Geometry check sheet. Reference: the model listing, model coordinates, mm. A direction names the side the tool comes from. Coordinates: 2 decimals unless noted, no trailing zeros. Write each loop counter-clockwise with the first axis right and the second up, starting at its lowest first coordinate (ties: lowest second). Pieces come first, ordered by that corner, then holes. Notation, with made-up numbers: (-2, -32.75) -> (36, -32.75) arc R24 cw to (36, 4.25) -> close; hole circle Ø6 at (87.25, 2). An arc over 180 degrees is marked (long way). Put each result on its own line as item: value. Start each with the question number.
from build123d import *
from OCP.BRepFilletAPI import BRepFilletAPI_MakeChamfer

# Parameters (mm, degrees)
SKETCH1_W           = 42
SKETCH1_H           = 130
BOSS_EXTRUDE1_DEPTH = 3
SKETCH2_W           = 27
SKETCH2_H           = 100
CUT_EXTRUDE1_DEPTH  = 3
BOSS_EXTRUDE2_DEPTH = 10
CHAMFER1_SIZE       = 43.314758743
CHAMFER1_SIZE_2     = 10
SKETCH5_R           = 1.75
CUT_EXTRUDE2_DEPTH  = 10
SKETCH6_W           = 7.5
SKETCH6_H           = 3
BOSS_EXTRUDE3_DEPTH = 10
LPATTERN1_COUNT     = 2
LPATTERN1_PITCH     = 10
FILLET1_R           = 10


with BuildPart() as part:
    # Sketch1 → Boss-Extrude1 (new body)
    with BuildSketch(Plane.XY):
        Rectangle(SKETCH1_W, SKETCH1_H)
    extrude(amount=BOSS_EXTRUDE1_DEPTH)

    # Sketch2 → Cut-Extrude1 (cut)
    with BuildSketch(Plane.XY.offset(3)):
        with Locations((0, -65)):
            Rectangle(SKETCH2_W, SKETCH2_H)
    extrude(amount=-CUT_EXTRUDE1_DEPTH, mode=Mode.SUBTRACT)

    # Sketch3 → Boss-Extrude2 (add)
    with BuildSketch(Plane(origin=(0, 0, 0), x_dir=(-1, 0, 0), z_dir=(0, 0, -1))):
        Polygon((-21, -65), (-13.5, -65), (-13.5, -62), (-13.5, -17), (-15.5, -17), (-15.5, -62), (-21, -62), align=None)
        Polygon((13.5, -65), (21, -65), (21, -62), (15.5, -62), (15.5, -17), (13.5, -17), (13.5, -62), align=None)
    extrude(amount=BOSS_EXTRUDE2_DEPTH)

    # Chamfer1
    chamfer1_edges_1 = [part.edges().sort_by_distance(p)[0] for p in [
        (-14.5, -17, -10),
    ]]
    chamfer1_side_1 = [part.faces().sort_by_distance(p)[0] for p in [
        (-14.5, -17.2, -10),
    ]]
    chamfer1_edges_2 = [part.edges().sort_by_distance(p)[0] for p in [
        (14.5, -17, -10),
    ]]
    chamfer1_side_2 = [part.faces().sort_by_distance(p)[0] for p in [
        (14.5, -17.2, -10),
    ]]
    chamfer1 = BRepFilletAPI_MakeChamfer(part.part.solid().wrapped)
    for e in chamfer1_edges_1:
        chamfer1.Add(CHAMFER1_SIZE - 0.0001, CHAMFER1_SIZE_2 - 0.0001, e.wrapped, chamfer1_side_1[0].wrapped)
    for e in chamfer1_edges_2:
        chamfer1.Add(CHAMFER1_SIZE - 0.0001, CHAMFER1_SIZE_2 - 0.0001, e.wrapped, chamfer1_side_2[0].wrapped)
    add(Compound.cast(chamfer1.Shape()), mode=Mode.REPLACE)  # a hair under: the kernel refuses the full size

    # Sketch5 → Cut-Extrude2 (cut)
    with BuildSketch(Plane.XZ.offset(65)):
        with Locations(Location((-17.5, -4.36859694, 0), (0, 0, 270))):
            Circle(SKETCH5_R)
        with Locations(Location((17.5, -4.36859694, 0), (0, 0, 270))):
            Circle(SKETCH5_R)
    cut_extrude2 = extrude(amount=-CUT_EXTRUDE2_DEPTH, mode=Mode.SUBTRACT)

    # Sketch6 → Boss-Extrude3 (add)
    with BuildSketch(Plane(origin=(0, 0, -10), x_dir=(-1, 0, 0), z_dir=(0, 0, -1))):
        with Locations((17.25, -63.5)):
            Rectangle(SKETCH6_W, SKETCH6_H)
        with Locations((-17.25, -63.5)):
            Rectangle(SKETCH6_W, SKETCH6_H)
    extrude(amount=BOSS_EXTRUDE3_DEPTH)

    # LPattern1: Cut-Extrude2 ×2
    with Locations(*[(0, 0, -i * LPATTERN1_PITCH) for i in range(1, LPATTERN1_COUNT)]):
        add(cut_extrude2, mode=Mode.SUBTRACT)

    # Fillet1
    fillet1_edges = [part.edges().sort_by_distance(p)[0] for p in [
        (-21, 65, 1.5),
        (21, 65, 1.5),
    ]]
    fillet(fillet1_edges, radius=FILLET1_R)


solid = part.part
Item 1: Scan lines: line 1 along Z through (x, y) = (13.5, 0); line 2 along Z through (x, y) = (17, -64); line 3 along Y through (x, z) = (18, -11.5). Record each from-to range of solid material in increasing order. Write a range as [from, to].
Item 2: Mould release check, pull along X, two halves, no side actions. Record for faces 1 (the cylindrical face through (18.683, -63.521, -13.079)), 2 (the cylindrical face through (-18.15, 61.99, 1.52)), 3 (the flat face through (15.5, -44, -4)), 4 (the flat face through (-14.51, -38.35, -4.93)): released by +X, released by -X, zero draft, split by the parting line, or undercut.
Item 3: Section check D-D, the plane z = -15. Enter the section's corners in (x, y).
Item 4: Section check A-A, the plane y = -24.5. Enter the section's corners in (x, z).
Item 5: Section check B-B, the plane z = 1.75. Enter the section's corners in (x, y).
Item 6: Go/stop test with flat-tipped pins: P1, Ø2, axis at y = -30, z = -3.5, coming from the -X side; P2, Ø8, axis at x = 5.5, y = 34.5, coming from the -Z side; P3, Ø12, axis at y = -38, z = -10, coming from the +X side. Record where each tip stops, or that it passes through.
Item 7: Section check C-C, the plane x = -17.5. Enter the section's corners in (y, z), and give its area (3 significant figures).
Item 8: Access from +Z, -Z, +X, -X, +Y, -Y to the whole of each face (thin tool, end or side, straight path). Record for faces 5 (the flat face through (0, -15, 2)), 6 (the flat face through (-15.5, -45, -4)), 7 (the cylindrical face through (17.99, 62.15, 1.52)).
From the geometry:
1. line 1: [0, 3]
1. line 2: [-20, -16.05], [-12.69, -6.05], [-2.69, 3]
1. line 3: [-65, -62]
2. face 1: undercut
2. face 2: released by -X
2. face 3: released by +X
2. face 4: zero draft
3. outline: (-21, -65) -> (-19.13, -65) -> (-19.13, -62) -> (-21, -62) -> close; (-15.87, -65) -> (-13.5, -65) -> (-13.5, -62) -> (-15.87, -62) -> close; (13.5, -65) -> (15.87, -65) -> (15.87, -62) -> (13.5, -62) -> close; (19.13, -65) -> (21, -65) -> (21, -62) -> (19.13, -62) -> close
4. outline: (-21, 0) -> (-15.5, 0) -> (-15.5, -1.73) -> (-13.5, -1.73) -> (-13.5, 3) -> (-21, 3) -> close; (13.5, -1.73) -> (15.5, -1.73) -> (15.5, 0) -> (21, 0) -> (21, 3) -> (13.5, 3) -> close
5. outline: (-21, -65) -> (-13.5, -65) -> (-13.5, -15) -> (13.5, -15) -> (13.5, -65) -> (21, -65) -> (21, 55) arc R10 ccw to (11, 65) -> (-11, 65) arc R10 ccw to (-21, 55) -> close
6. P1: x = -15.5
6. P2: z = 0
6. P3: x = 15.5
7. outline: (-65, -20) -> (-62, -20) -> (-62, -16.12) -> (-65, -16.12) -> close; (-65, -12.62) -> (-62, -12.62) -> (-62, -6.12) -> (-65, -6.12) -> close; (-65, -2.62) -> (-62, -2.62) -> (-62, 0) -> (62.6, 0) -> (62.6, 3) -> (-65, 3) -> close
7. area: 422 mm²
8. face 5: +Z, -Z, -Y
8. face 6: -Z, -X, +Y
8. face 7: +Z, -Z, +X, +Y
